Geometry: see drawing. Coordinates: mm, zero at the bounding-box minimum. A direction names the side the tool comes from. Give positions to 0.01 mm unless a question says otherwise; leave off trailing zeros. Write each loop counter-clockwise with the first axis right and the second up, starting at its lowest first coordinate (ties: lowest second). Pieces come first, ordered by that corner, then holes. Notation, with made-up numbers: M -8,-25.75 L 28,-25.75 A19 ccw 28,-20.75 Z; hole C -1.75,7.5 d1. An arc over 180 degrees is marked long. Answer as a JSON object with one key per item and string values. Group by question number.
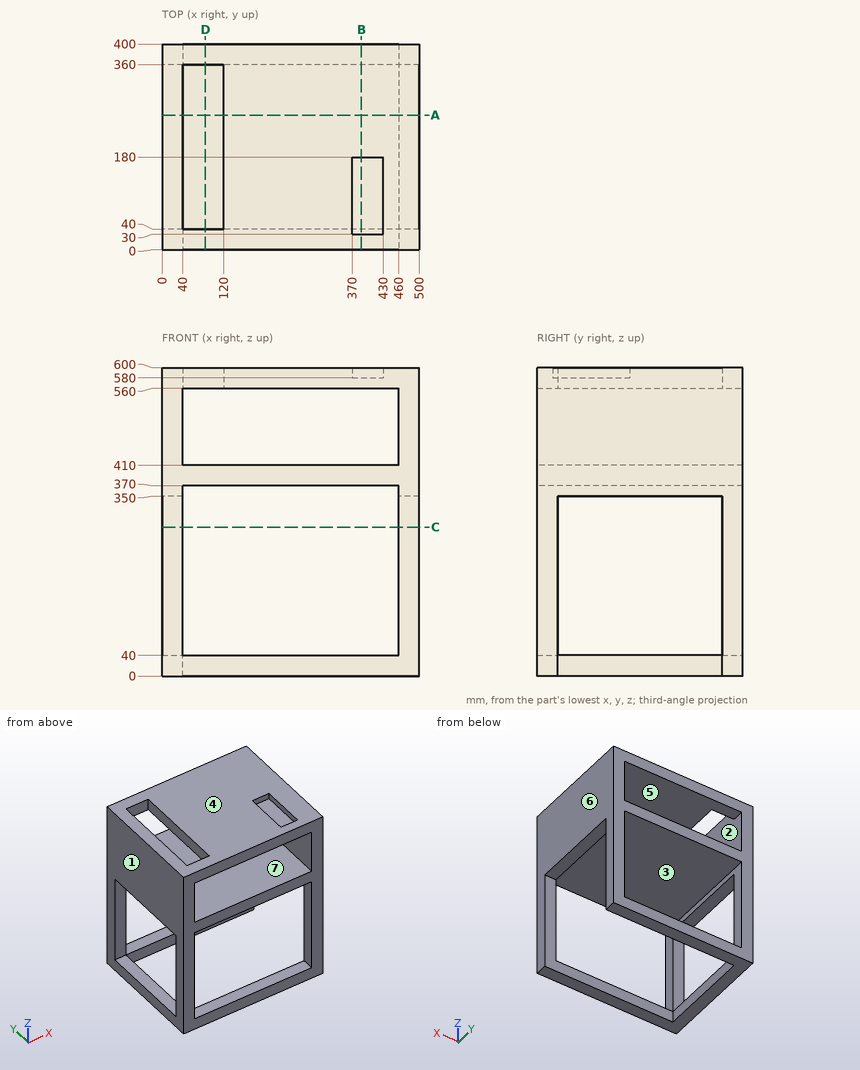
(1) Section B-B, the plane x = 387.5. Return loops of the section in (y, z).
(2) Contact query for flat-ended pins moving along their axis: pin 1 Ø18 at (x, y) = (397, 88.5) entering from +Z; pin 2 Ø6 at (x, y) = (96.5, 105) entering from +Z. Output: stop coordinate, or through.
(3) Section D-D, the plane x = 84. Return loops of the section in (y, z), plus the area to 3 significant figures.
(4) Section A-A, the plane y = 261.5. Return loops of the section in (x, z).
(5) Ray query, L1, parallel to Z at x = 117.5, y = 22.5; L2, parallel to Z at x = 381.5, y = 251; L3, parallel to Y at x = 92, z = 563.5. Return the intervals inside material, ascending. Write a range as [from, to].
(6) Pull-direction query (Z, two-part tool) for the marked faces 4, 5, 6 and 7; classes: pulls with the +Z half, pulls with the -Z half, needs draft (parallel to the pull), parting line crosses it, or undercut.
(7) Access query for the marked faces 1, 2 and 3. Directions: +Z, -Z, +X, -X, +Y, -Y. A direction counts if a zero-diameter tool reaches every point of the face in a straight line with its end or side. Return the directions, or none.
(8) Section C-C, the plane z = 289.5. Return loops of the section in (x, y), plus the area to 3 significant figures.
Reported:
{
 "1": {"outline": "M 0,0 L 40,0 L 40,40 L 0,40 Z; M 0,370 L 400,370 L 400,410 L 0,410 Z; M 0,560 L 400,560 L 400,600 L 180,600 L 180,580 L 30,580 L 30,600 L 0,600 Z; M 360,0 L 400,0 L 400,40 L 360,40 Z"},
 "2": {"pin 1": "stops at z = 580", "pin 2": "stops at z = 410"},
 "3": {"outline": "M 0,0 L 40,0 L 40,40 L 0,40 Z; M 0,370 L 400,370 L 400,410 L 0,410 Z; M 0,560 L 40,560 L 40,600 L 0,600 Z; M 360,0 L 400,0 L 400,40 L 360,40 Z; M 360,560 L 400,560 L 400,600 L 360,600 Z", "area": "22,400 mm2"},
 "4": {"outline": "M 0,0 L 40,0 L 40,40 L 0,40 Z; M 0,350 L 40,350 L 40,370 L 460,370 L 460,350 L 500,350 L 500,600 L 120,600 L 120,560 L 460,560 L 460,410 L 40,410 L 40,600 L 0,600 Z"},
 "5": {"L1": "z = [0, 40], [370, 410], [560, 600]", "L2": "z = [370, 410], [560, 600]", "L3": "y = [0, 40], [360, 400]"},
 "6": {"face 4": "pulls with the +Z half", "face 5": "undercut", "face 6": "needs draft", "face 7": "undercut"},
 "7": {"face 1": "+Z, -Z, -X, +Y, -Y", "face 2": "none", "face 3": "+Y, -Y"},
 "8": {"outline": "M 0,0 L 40,0 L 40,40 L 0,40 Z; M 0,360 L 40,360 L 40,400 L 0,400 Z; M 460,0 L 500,0 L 500,40 L 460,40 Z; M 460,360 L 500,360 L 500,400 L 460,400 Z", "area": "6,400 mm2"}
}
